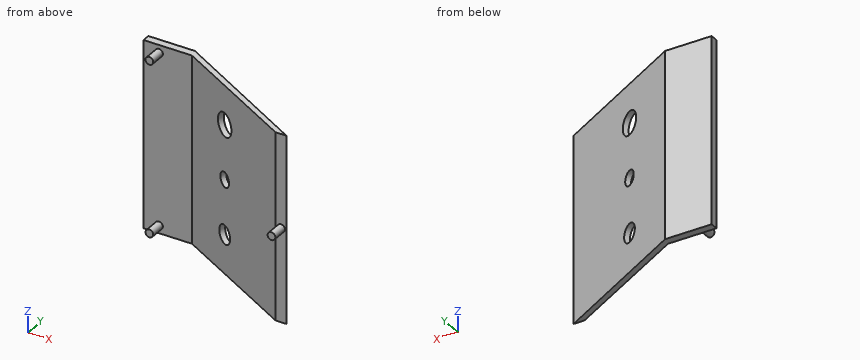
```python
from build123d import *

# Parameters (mm, degrees)
SKETCH1_W           = 152.4
SKETCH1_H           = 76.2
BOSS_EXTRUDE1_DEPTH = 152.4
CUT_EXTRUDE1_DEPTH  = 152.4
CUT_EXTRUDE4_DEPTH  = 152.4
SKETCH6_R           = 9.525
SKETCH6_R_2         = 6.096
SKETCH6_R_3         = 7.62
CUT_EXTRUDE5_DEPTH  = 25.4
SKETCH7_R           = 3.175
BOSS_EXTRUDE2_DEPTH = 12.7
SKETCH8_W           = 9.01836237
SKETCH8_H           = 12.7
CUT_EXTRUDE6_DEPTH  = 152.4
SKETCH9_R           = 3.175
BOSS_EXTRUDE3_DEPTH = 12.7


with BuildPart() as part:
    # Sketch1 → Boss-Extrude1 (new body)
    with BuildSketch(Plane.XY):
        with Locations((76.2, 38.1)):
            Rectangle(SKETCH1_W, SKETCH1_H)
    extrude(amount=BOSS_EXTRUDE1_DEPTH)

    # Sketch2 → Cut-Extrude1 (cut)
    with BuildSketch(Plane.XY.offset(152.4)):
        Polygon((152.4, 76.2), (38.1, 76.2), (152.4, 12.7), align=None)
    extrude(amount=-CUT_EXTRUDE1_DEPTH, mode=Mode.SUBTRACT)

    # Sketch4 → Cut-Extrude4 (cut)
    with BuildSketch(Plane.XY.offset(152.4)):
        Polygon((39.625354208, 69.85), (146.05, 11.230239284), (146.05, 0), (0, 0), (0, 69.85), align=None)
    extrude(amount=-CUT_EXTRUDE4_DEPTH, mode=Mode.SUBTRACT)

    # Sketch6 → Cut-Extrude5 (cut)
    with BuildSketch(Plane(origin=(41.33490566, 74.402830189, 0), x_dir=(0.874157276, -0.485642931, 0), z_dir=(0.485642931, 0.874157276, 0))):
        with Locations((47.099400864, -120.65)):
            Circle(SKETCH6_R)
        with Locations((47.099400864, -76.2)):
            Circle(SKETCH6_R_2)
        with Locations((47.099400864, -31.75)):
            Circle(SKETCH6_R_3)
    extrude(amount=-CUT_EXTRUDE5_DEPTH, mode=Mode.SUBTRACT)

    # Sketch7 → Boss-Extrude2 (add)
    with BuildSketch(Plane.XZ.offset(-69.85)):
        with Locations((12.7, 6.35)):
            Circle(SKETCH7_R)
        with Locations((12.7, 146.05)):
            Circle(SKETCH7_R)
    extrude(amount=BOSS_EXTRUDE2_DEPTH)

    # Sketch8 → Cut-Extrude6 (cut)
    with BuildSketch(Plane.XY.offset(152.4)):
        with Locations((147.890818815, 6.35)):
            Rectangle(SKETCH8_W, SKETCH8_H)
    extrude(amount=-CUT_EXTRUDE6_DEPTH, mode=Mode.SUBTRACT)

    # Sketch9 → Boss-Extrude3 (add)
    with BuildSketch(Plane.XZ.offset(-12.7)):
        with Locations((147.955, 76.2)):
            Circle(SKETCH9_R)
    extrude(amount=BOSS_EXTRUDE3_DEPTH)


solid = part.part
```
CAD build for the part. Positions are in the model's coordinates, mm. Round coordinates to 2 decimals unless told otherwise and drop trailing zeros. Order: outer loops, then holes, each group sorted by start corner. A loop starts at its lowest first (then second) coordinate and runs counter-clockwise, first axis right, second up. Notation, with made-up numbers: (72.25, 60.5) -> (114.25, 60.5) arc R21 cw to (114.25, 70.5) -> close; hole circle Ø3 at (7.5, -18.5). An arc over 180 degrees is marked (long way). One line per question, with ' | ' between items.
Q1. Drop flat-ended pins along their axis: pin 1 (1 mm diameter, centred on x = 136, z = 119.5, fed in from +Y); pin 2 (3 mm diameter, centred on x = 14, z = 7, fed in from -Y); pin 3 (3 mm diameter, centred on y = 11.5, z = 57, fed in from +X). Give the stop position or say it passes through.
Completed:
pin 1: stops at y = 22.09 | pin 2: stops at y = 57.15 | pin 3: stops at x = 152.4
Q2. Slice it at A-A (x = 12.7). Write the cut outline in (y, z) (3 decimals), then the cut area to 3 significant figures.
Completed:
outline: (57.15, 3.175) -> (69.85, 3.175) -> (69.85, 0) -> (76.2, 0) -> (76.2, 152.4) -> (69.85, 152.4) -> (69.85, 149.225) -> (57.15, 149.225) -> (57.15, 142.875) -> (69.85, 142.875) -> (69.85, 9.525) -> (57.15, 9.525) -> close | area: 1,130 mm^2
Q3. Slice it at D-D (x = 80.5). Give the number of separate pieces and of enclosed holes in the cut face, then the cut area to 3 significant figures.
Completed:
separate pieces: 4 | enclosed holes: 0 | area: 566 mm^2
Q4. Slice it at C-C (z = 6.35). Write the cut outline in (x, y) (3 decimals), then the cut area to 3 significant figures.
Completed:
outline: (0, 69.85) -> (9.525, 69.85) -> (9.525, 57.15) -> (15.875, 57.15) -> (15.875, 69.85) -> (39.625, 69.85) -> (143.382, 12.7) -> (152.4, 12.7) -> (38.1, 76.2) -> (0, 76.2) -> close | area: 900 mm^2
Q5. Probe probe 1 along Y at (x, z) = (13.5, 112.5); probe 2 along X at (y, z) = (59, 10); probe 3 along X at (y, z) = (58, 80). List the from-to ranges inside material, lowest first.
Completed:
probe 1: y = 69.85 to 76.2 | probe 2: x = 59.32 to 69.06 | probe 3: x = 61.14 to 70.86
Q6. Slice it at B-B (z = 125). Write the cut outline in (x, y), then the cut area to 3 significant figures.
Completed:
outline: (0, 69.85) -> (39.63, 69.85) -> (72.83, 51.56) -> (75.1, 55.64) -> (38.1, 76.2) -> (0, 76.2) -> close; (87.68, 43.38) -> (143.38, 12.7) -> (152.4, 12.7) -> (89.91, 47.41) -> close | area: 740 mm^2
